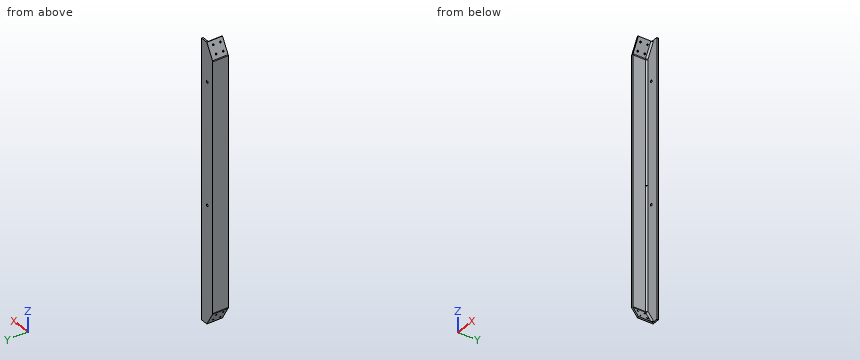
```python
from build123d import *

# Parameters (mm, degrees)
BOSS_EXTRUDE1_DEPTH  = 640
BOSS_EXTRUDE2_DEPTH  = 8
BOSS_EXTRUDE3_DEPTH  = 72
SKETCH6_R            = 4
CUT_EXTRUDE1_DEPTH   = 8
FILLET1_R            = 10
FILLET2_R            = 8
FILLET1_OF_MIRROR1_R = 10
FILLET2_OF_MIRROR1_R = 8
SKETCH8_R            = 6
CUT_EXTRUDE2_DEPTH   = 8


with BuildPart() as part:
    # Sketch1 → Boss-Extrude1 (new body)
    with BuildSketch(Plane.XY):
        Polygon((-8, 8), (72, 8), (72, 0), (0, 0), (0, -72), (-8, -72), align=None)
    boss_extrude1 = extrude(amount=BOSS_EXTRUDE1_DEPTH)

    # Sketch3 → Boss-Extrude2 (add)
    with BuildSketch(Plane(origin=(0, 0, 0), x_dir=(1, 0, 0), z_dir=(0, 1, 0))):
        Polygon((-8, -640), (34.5, -713.612159322), (72, -713.612159322), (72, -640), align=None)
    boss_extrude2 = extrude(amount=BOSS_EXTRUDE2_DEPTH)

    # Sketch4 → Boss-Extrude3 (add)
    with BuildSketch(Plane.XZ):
        Polygon((-8, 640), (34.5, 713.612159322), (40.5, 710.148057707), (0, 640), align=None)
    boss_extrude3 = extrude(amount=BOSS_EXTRUDE3_DEPTH)

    # Sketch6 → Cut-Extrude1 (cut)
    with BuildSketch(Plane(origin=(-277.128129211, 0, 160), x_dir=(-0.4999999999999956, 0, -0.8660254037844413), z_dir=(0.8660254037844413, 0, -0.4999999999999956))):
        with Locations((-615.006258422, -18)):
            Circle(SKETCH6_R)
        with Locations((-574.506258422, -18)):
            Circle(SKETCH6_R)
        with Locations((-574.506258422, -54)):
            Circle(SKETCH6_R)
        with Locations((-615.006258422, -54)):
            Circle(SKETCH6_R)
    cut_extrude1 = extrude(amount=-CUT_EXTRUDE1_DEPTH, mode=Mode.SUBTRACT)

    # Fillet1
    fillet1_edges = [part.edges().sort_by_distance(p)[0] for p in [
        (0, -36, 640),
        (-8, -32, 640),
    ]]
    fillet(fillet1_edges, radius=FILLET1_R)

    # Fillet2
    fillet2_edges = [part.edges().sort_by_distance(p)[0] for p in [
        (20.919872981, 0, 676.234282891),
        (0, 0, 318.660254038),
        (0.340741737, 0, 639.908698527),
    ]]
    fillet(fillet2_edges, radius=FILLET2_R)

    # Mirror1: Boss-Extrude1, Boss-Extrude2, Boss-Extrude3, Cut-Extrude1 across plane
    add(boss_extrude1.mirror(Plane.XY))
    add(boss_extrude2.mirror(Plane.XY))
    add(boss_extrude3.mirror(Plane.XY))
    add(cut_extrude1.mirror(Plane.XY), mode=Mode.SUBTRACT)

    # Fillet1 of Mirror1
    fillet1_of_mirror1_edges = [part.edges().sort_by_distance(p)[0] for p in [
        (0, -36, -640),
        (-8, -32, -640),
    ]]
    fillet(fillet1_of_mirror1_edges, radius=FILLET1_OF_MIRROR1_R)

    # Fillet2 of Mirror1
    fillet2_of_mirror1_edges = [part.edges().sort_by_distance(p)[0] for p in [
        (20.919872981, 0, -676.234282891),
        (0, 0, -318.660254038),
        (0.340741737, 0, -639.908698527),
    ]]
    fillet(fillet2_of_mirror1_edges, radius=FILLET2_OF_MIRROR1_R)

    # Sketch8 → Cut-Extrude2 (cut)
    with BuildSketch(Plane(origin=(0, 8, 0), x_dir=(1, 0, 0), z_dir=(0, 1, 0))):
        with Locations(Location((32, 111.387840678, 0), (0, 0, 180))):
            Circle(SKETCH8_R)
        with Locations(Location((32, -513.612159322, 0), (0, 0, 180))):
            Circle(SKETCH8_R)
    extrude(amount=-CUT_EXTRUDE2_DEPTH, mode=Mode.SUBTRACT)


solid = part.part
```
Build history of the part. All positions in model axes, mm. Round coordinates to 2 decimals unless told otherwise and drop trailing zeros. Order: outer loops, then holes, each group sorted by start corner. A loop starts at its lowest first (then second) coordinate and runs counter-clockwise, first axis right, second up. Notation, with made-up numbers: (16, 4.5) -> (60, 4.5) arc R24 cw to (60, 30.5) -> close; hole circle Ø4 at (83, 53.5). An arc over 180 degrees is marked (long way). Answer in a Markdown table with one row per item.
1) Pin check, flat tips, straight feed: P1, Ø3, axis at x = 58.5, z = 330.5, coming from the -Y side; P2, Ø4, axis at x = 34, y = -5.5, coming from the +Z side; P3, Ø2.5, axis at x = 4, y = -2, coming from the -Z side. Stop position of each tip, or through.
Values:
| item | result |
|---|---|
| P1 | y = 0 |
| P2 | z = 713.61 |
| P3 | z = -662.95 |
2) Band-saw the part on B-B on x = 59. Give the cut face in (y, z), and give its area (3 significant figures).
Values:
| item | result |
|---|---|
| outline | (0, -713.61) -> (8, -713.61) -> (8, 713.61) -> (0, 713.61) -> close |
| area | 11,400 mm2 |
3) Wall check: L1, parallel to Z at x = 32, y = 4; L2, parallel to X at y = -13, z = 515; L3, parallel to Y at x = 44.5, z = -46.5. Give the ranges that are in metal, low to high.
Values:
| item | result |
|---|---|
| L1 | -709.28 to -117.39, -105.39 to 507.61, 519.61 to 709.28 |
| L2 | -8 to 0 |
| L3 | 0 to 8 |
4) Band-saw the part on A-A on z = 83. Give the cut face in (x, y).
Values:
| item | result |
|---|---|
| outline | (-8, -72) -> (0, -72) -> (0, -8) arc R8 cw to (8, 0) -> (72, 0) -> (72, 8) -> (-8, 8) -> close |
